Read the model definition and answer for the solid it produces. Units are mm, in the model's axes. Give positions to 0.01 mm unless a question says otherwise; leave off trailing zeros. Order: outer loops, then holes, each group sorted by start corner. A loop starts at its lowest first (then second) coordinate and runs counter-clockwise, first axis right, second up. Notation, with made-up numbers: (-23.5, -18.75) - (35.5, -18.75) arc R27 cw to (35.5, 9.25) - close; hole circle Ø5 at (80.5, -8.5). An arc over 180 degrees is marked (long way). Write item = value, one per line.
Autodesk Inventor part; units mm, degrees
ref_plane "YZ Plane" through (0, 0, 0) normal (1, 0, 0) x (0, 1, 0)
ref_plane "XZ Plane" through (0, 0, 0) normal (0, 1, 0) x (-1, 0, 0)
ref_plane "XY Plane" through (0, 0, 0) normal (0, 0, 1) x (1, 0, 0)
sketch "Sketch6" plane through (0, 0, 0) normal (0, 1, 0) x (-1, 0, 0)
  line L0 (255.9, -990) -> (-255.9, -990)
  line L1 (-255.9, -990) -> (-255.9, 990)
  line L2 (-255.9, 990) -> (255.9, 990)
  line L3 (255.9, 990) -> (255.9, -990)
  line L4 (255.9, -990) -> (-255.9, 990) construction
  line L5 (-255.9, -990) -> (255.9, 990) construction
  point P0 (0, 0)
  dimension "d52" = 511.8
  dimension "d53" = 1980
extrude "Plate2" add sketch "Sketch6" along normal blind 0.5
sketch "Sketch12" plane through (255.4, 0, -990) normal (1, 0, 0) x (0, 1, 0)
  line L0 (0, 1980) -> (0, 0)
  line L1 (0, 0) -> (10, 0)
  line L2 (10, 0) -> (10, 1980)
  line L3 (10, 1980) -> (0, 1980)
edge flange "Flange3" height 10 angle 90 thickness 0.5 bend radius 0.5 thickness toward (1, 0, 0) relief tear relief width 0.5 relief depth 0.25 edges at (255.9, 0.5, 0) wall of the first edge with corners at (255.4, 0, 990) (255.4, 0, -990) (255.4, 10, -990) (255.4, 10, 990)
bend "Bend4"
corner "Corner4"
sketch "Sketch13" plane through (255.9, 9.5, -990) normal (0, 1, 0) x (-1, 0, 0)
  line L0 (0, 1980) -> (0, 0)
  line L1 (0, 0) -> (10, 0)
  line L2 (10, 0) -> (10, 1980)
  line L3 (10, 1980) -> (0, 1980)
edge flange "Flange4" height 10 angle 90 thickness 0.5 bend radius 0.5 thickness toward (0, 1, 0) relief tear relief width 0.5 relief depth 0.25 edges at (255.4, 10, 0) wall of the first edge with corners at (255.9, 9.5, 990) (255.9, 9.5, -990) (245.9, 9.5, -990) (245.9, 9.5, 990)
bend "Bend5"
corner "Corner5"
sketch "Sketch14" plane through (-255.4, 0, 990) normal (-1, 0, 0) x (0, -1, 0)
  line L0 (0, -1980) -> (0, 0)
  line L1 (0, 0) -> (-10, 0)
  line L2 (-10, 0) -> (-10, -1980)
  line L3 (-10, -1980) -> (0, -1980)
edge flange "Flange5" height 10 angle 90 thickness 0.5 bend radius 0.5 thickness toward (-1, 0, 0) relief tear relief width 0.5 relief depth 0.25 edges at (-255.9, 0.5, 0) wall of the first edge with corners at (-255.4, 0, -990) (-255.4, 0, 990) (-255.4, 10, 990) (-255.4, 10, -990)
bend "Bend6"
corner "Corner6"
sketch "Sketch15" plane through (-255.9, 9.5, 990) normal (0, 1, 0) x (-1, 0, 0)
  line L0 (0, -1980) -> (0, 0)
  line L1 (0, 0) -> (-10, 0)
  line L2 (-10, 0) -> (-10, -1980)
  line L3 (-10, -1980) -> (0, -1980)
edge flange "Flange6" height 10 angle 90 thickness 0.5 bend radius 0.5 thickness toward (0, 1, 0) relief tear relief width 0.5 relief depth 0.25 edges at (-255.4, 10, 0) wall of the first edge with corners at (-255.9, 9.5, -990) (-255.9, 9.5, 990) (-245.9, 9.5, 990) (-245.9, 9.5, -990)
bend "Bend7"
corner "Corner7"
equation "\"d52\" = ЖАБРЫ_базовая_ширина - 4 * ЖАБРЫ_шаг_листов"
equation "\"d53\" = ЖАБРЫ_базовая_длина_дл_лист"
equation "\"d54\" = Thickness"
equation "\"d94\" = BendReliefWidth"
equation "\"d95\" = BendReliefDepth"
equation "\"d96\" = MinimumRemnant"
equation "\"d97\" = TransitionRadius"
equation "\"d100\" = BendRadius"
equation "\"d101\" = CornerReliefSize"
equation "\"d102\" = GapSize"
equation "\"d103\" = JacobiRadiusSize"
equation "\"d104\" = BendReliefWidth"
equation "\"d105\" = BendReliefDepth"
equation "\"d106\" = MinimumRemnant"
equation "\"d107\" = TransitionRadius"
equation "\"d110\" = BendRadius"
equation "\"d111\" = CornerReliefSize"
equation "\"d112\" = GapSize"
equation "\"d113\" = JacobiRadiusSize"
equation "\"d114\" = BendReliefWidth"
equation "\"d115\" = BendReliefDepth"
equation "\"d116\" = MinimumRemnant"
equation "\"d117\" = TransitionRadius"
equation "\"d120\" = BendRadius"
equation "\"d121\" = CornerReliefSize"
equation "\"d122\" = GapSize"
equation "\"d123\" = JacobiRadiusSize"
equation "\"d124\" = BendReliefWidth"
equation "\"d125\" = BendReliefDepth"
equation "\"d126\" = MinimumRemnant"
equation "\"d127\" = TransitionRadius"
equation "\"d130\" = BendRadius"
equation "\"d131\" = CornerReliefSize"
equation "\"d132\" = GapSize"
equation "\"d133\" = JacobiRadiusSize"
equation "\"BendRadius\" = Thickness"
equation "\"BendReliefWidth\" = Thickness"
equation "\"BendReliefDepth\" = 0.5 * Thickness"
equation "\"CornerReliefSize\" = 4 * Thickness"
equation "\"MinimumRemnant\" = 2 * Thickness"
equation "\"TransitionRadius\" = BendRadius"
equation "\"JacobiRadiusSize\" = BendRadius"
equation "\"GapSize\" = Thickness"
properties part number "MSC 810 sheet gills" material "Stainless Steel"
1. Determine the mould class of faces 1 (the face through (4, 0, 14)), 2 (the face through (4, 0.5, 14)) for opening direction X: +X half, -X half, draft (parallel to the pull), parting line (faces both ways), or undercut.
Recorded:
face_1 = draft
face_2 = undercut
2. Flat-ended cylindrical pins translate along their axes: pin 1 (7 mm diameter, centred on x = 249, z = -31, fed in from -Y); pin 2 (12 mm diameter, centred on x = -122.5, z = 498, fed in from +Y). Find the tip coordinate at first contact, or state that the pin passes through.
Recorded:
pin_1 = 0
pin_2 = 0.5
3. Section B-B (z = 665.5) is taken. Determine the outline of the cut face in (x, y), and give its area (3 significant figures).
Recorded:
outline = (-255.9, 1) arc R1 ccw to (-254.9, 0) - (254.9, 0) arc R1 ccw to (255.9, 1) - (255.9, 9) arc R1 ccw to (254.9, 10) - (245.9, 10) - (245.9, 9.5) - (254.9, 9.5) arc R0.5 cw to (255.4, 9) - (255.4, 1) arc R0.5 cw to (254.9, 0.5) - (-254.9, 0.5) arc R0.5 cw to (-255.4, 1) - (-255.4, 9) arc R0.5 cw to (-254.9, 9.5) - (-245.9, 9.5) - (-245.9, 10) - (-254.9, 10) arc R1 ccw to (-255.9, 9) - close
area = 274 mm^2
4. Straight lines are drawn through the part: L1, parallel to X at y = 6.75, z = -278.5; L2, parallel to Y at x = 214.5, z = 708.5. For each, find the intervals that lie inside material, in ascending order. Write a range as [from, to].
Recorded:
L1 = [-255.9, -255.4], [255.4, 255.9]
L2 = [0, 0.5]
5. Section C-C (x = 59) is taken. Determine the outline of the cut face in (y, z).
Recorded:
outline = (0, -990) - (0.5, -990) - (0.5, 990) - (0, 990) - close
6. Section A-A (y = 4.5) is taken. Determine the outline of the cut face in (x, z).
Recorded:
outline = (-255.9, -990) - (-255.4, -990) - (-255.4, 990) - (-255.9, 990) - close; (255.4, -990) - (255.9, -990) - (255.9, 990) - (255.4, 990) - close
